Build history of the part. All positions in model axes, mm. Face numbers are marked on the shaded views. A direction names the side the tool comes from. Coordinates: 2 decimals unless noted, no trailing zeros. Order: outer loops, then holes, each group sorted by start corner. A loop starts at its lowest first (then second) coordinate and runs counter-clockwise, first axis right, second up. Notation, with made-up numbers: (28, 35) - (35, 35) arc R15 ccw to (35, 45) - close; hole circle Ø8 at (-40, 2.5). An arc over 180 degrees is marked (long way). One line per item, written item: value.
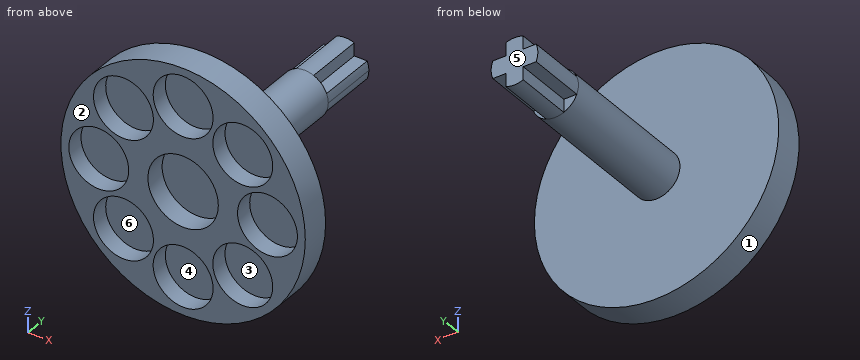
from build123d import *

# Parameters (mm, degrees)
SKETCH_1_R               = 21
EXTRUDE_1_DEPTH          = 5
SKETCH_3_R               = 6.05
CUT_EXTRUDE_2_DEPTH      = 3.5
SKETCH_4_R               = 4.015
EXTRUDE_2_DEPTH          = 25
SKETCH_12_R              = 5.15
CUT_EXTRUDE_6_DEPTH      = 3
PATTERN_CIRCULAR_1_COUNT = 8
SKETCH_13_W              = 3
SKETCH_13_H              = 3
EXTRUDE_3_DEPTH          = 10


with BuildPart() as part:
    # 스케치1 → 보스-돌출1 (new body)
    with BuildSketch(Plane(origin=(0, 0, 0), x_dir=(1, 0, 0), z_dir=(0, 1, 0))):
        Circle(SKETCH_1_R)
    extrude(amount=EXTRUDE_1_DEPTH)

    # 스케치3 → 컷-돌출2 (cut)
    with BuildSketch(Plane.XZ):
        Circle(SKETCH_3_R)
    extrude(amount=-CUT_EXTRUDE_2_DEPTH, mode=Mode.SUBTRACT)

    # 스케치4 → 보스-돌출2 (add)
    with BuildSketch(Plane(origin=(0, 5, 0), x_dir=(1, 0, 0), z_dir=(0, 1, 0))):
        Circle(SKETCH_4_R)
    extrude(amount=EXTRUDE_2_DEPTH)

    # 스케치12 → 컷-돌출6 (cut)
    with BuildSketch(Plane.XZ):
        with Locations((0, -14.5)):
            Circle(SKETCH_12_R)
    cut_extrude_6 = extrude(amount=-CUT_EXTRUDE_6_DEPTH, mode=Mode.SUBTRACT)

    # 원형 패턴1: 컷-돌출6 ×8 about axis
    pattern_circular_1_axis = Axis((0, 0, 0), (0, 1, 0))
    for i in range(1, PATTERN_CIRCULAR_1_COUNT):
        add(cut_extrude_6.rotate(pattern_circular_1_axis, i * 360 / PATTERN_CIRCULAR_1_COUNT), mode=Mode.SUBTRACT)

    # 스케치13 → 보스-돌출3 (add)
    with BuildSketch(Plane(origin=(0, 30, 0), x_dir=(1, 0, 0), z_dir=(0, 1, 0))):
        with BuildLine():
            ThreePointArc((1.5, 3.724275097), (0, 4.015), (-1.5, 3.724275097))
            Line((-1.5, 3.724275097), (-1.5, 1.5))
            Line((-1.5, 1.5), (1.5, 1.5))
            Line((1.5, 1.5), (1.5, 3.724275097))
        make_face()
        with BuildLine():
            Line((-1.5, -1.5), (-1.5, 1.5))
            Line((-1.5, 1.5), (-3.724275097, 1.5))
            ThreePointArc((-3.724275097, 1.5), (-4.015, 0), (-3.724275097, -1.5))
            Line((-3.724275097, -1.5), (-1.5, -1.5))
        make_face()
        Rectangle(SKETCH_13_W, SKETCH_13_H)
        with BuildLine():
            Line((1.5, -1.5), (-1.5, -1.5))
            Line((-1.5, -1.5), (-1.5, -3.724275097))
            ThreePointArc((-1.5, -3.724275097), (0, -4.015), (1.5, -3.724275097))
            Line((1.5, -3.724275097), (1.5, -1.5))
        make_face()
        with BuildLine():
            Line((3.724275097, 1.5), (1.5, 1.5))
            Line((1.5, 1.5), (1.5, -1.5))
            Line((1.5, -1.5), (3.724275097, -1.5))
            ThreePointArc((3.724275097, -1.5), (3.941648736, -0.763956964), (4.015, 0))
            ThreePointArc((4.015, 0), (3.941648736, 0.763956964), (3.724275097, 1.5))
        make_face()
    extrude(amount=EXTRUDE_3_DEPTH)


solid = part.part
1. Band-saw the part on C-C, the plane z = 14.5. Give the cut face in (x, y).
Values found:
outline: (-15.19, 0) - (-13.17, 0) - (-13.17, 3) - (-7.34, 3) - (-7.34, 0) - (-5.15, 0) - (-5.15, 3) - (5.15, 3) - (5.15, 0) - (7.34, 0) - (7.34, 3) - (13.17, 3) - (13.17, 0) - (15.19, 0) - (15.19, 5) - (-15.19, 5) - close
2. Two-plate mould, pull along Z, no slides. Class the marked faces 1, 2, 3 and 4: pulls with the +Z half, pulls with the -Z half, needs draft (parallel to the pull), parting line crosses it, or undercut.
Values found:
face 1: parting line crosses it
face 2: needs draft
face 3: undercut
face 4: undercut
3. Band-saw the part on A-A, the plane y = 35. Give the cut face in (x, z) (3 decimals).
Values found:
outline: (-3.724, -1.5) - (-1.5, -1.5) - (-1.5, -3.724) arc R4.015 ccw to (1.5, -3.724) - (1.5, -1.5) - (3.724, -1.5) arc R4.015 ccw to (3.724, 1.5) - (1.5, 1.5) - (1.5, 3.724) arc R4.015 ccw to (-1.5, 3.724) - (-1.5, 1.5) - (-3.724, 1.5) arc R4.015 ccw to start
4. Band-saw the part on D-D, the plane x = 11.5. Give the cut face in (y, z), and give its area (3 significant figures).
Values found:
outline: (0, -17.57) - (5, -17.57) - (5, 17.57) - (0, 17.57) - (0, 15.25) - (3, 15.25) - (3, 5.26) - (0, 5.26) - (0, 4.19) - (3, 4.19) - (3, -4.19) - (0, -4.19) - (0, -5.26) - (3, -5.26) - (3, -15.25) - (0, -15.25) - close
area: 90.6 mm2
5. 3-axis set-ups, long thin cutter, end or side, ignore diameter. For the marked faces 5 and 6: which of +Z, -Z, +X, -X, +Y, -Y reach the whole face in a straight line?
Values found:
face 5: +Z, -Z, +X, -X, +Y
face 6: -Y
6. Band-saw the part on B-B, the plane x = 0. Give the cut face in (y, z) (3 decimals), and give its area (3 significant figures).
Values found:
outline: (0, -21) - (5, -21) - (5, -4.015) - (40, -4.015) - (40, 4.015) - (5, 4.015) - (5, 21) - (0, 21) - (0, 19.65) - (3, 19.65) - (3, 9.35) - (0, 9.35) - (0, 6.05) - (3.5, 6.05) - (3.5, -6.05) - (0, -6.05) - (0, -9.35) - (3, -9.35) - (3, -19.65) - (0, -19.65) - close
area: 387 mm2
7. Probe line 1 along Z through (x, y) = (0, 2); line 2 along Y through (x, z) = (-16, -2); line 3 along Y through (x, z) = (2.5, 1). List the from-to ranges inside material, lowest first.
Values found:
line 1: z = -21 to -19.65, -9.35 to -6.05, 6.05 to 9.35, 19.65 to 21
line 2: y = 3 to 5
line 3: y = 3.5 to 40
8. Flat gauge pins, fed straight in: P1, Ø1.1, axis at x = 3, z = 3, coming from the +Y side; P2, Ø1.5, axis at x = 14, z = 7.5, coming from the -Y side; P3, Ø8, axis at x = 0, z = 14.5, coming from the +Y side; P4, Ø2.5, axis at x = 2.5, y = 33.5, coming from the +Z side. Where does each tip first touch, or does it go through?
Values found:
P1: stops at y = 30
P2: stops at y = 0
P3: stops at y = 5
P4: stops at z = 3.82
